Model file for the job. Use its own axes, mm. A direction names the side the tool comes from. Round coordinates to 2 decimals unless told otherwise and drop trailing zeros. Loops run counter-clockwise (first coordinate to the right, second up) from the corner with the lowest first, then second, coordinate; pieces in that order, holes last. Notation, with made-up numbers: M 32.5,49.25 L 82.5,49.25 A29 ccw 82.5,85.25 Z; hole C 2.25,19.5 d6. An arc over 180 degrees is marked long. Use a Markdown table: item, result. Add a question column.
Q1. Mould opens along X. For faces 1 (the face through (-10.867, 76.095, 2.958)), 2 (the face through (-3, 4, 3)), 3 (the face through (-10, 46, 0)) say: +X half, -X half, draft (parallel to the pull), parting line (faces both ways), or undercut.
Q2. Cut at D-D (y = 21). Give the cut face in (x, z).
Q3. Cut at B-B (z = 3.75). Give the cut face in (x, y), plus the area to 3 significant figures.
Q4. Tool access for faces 4 (the face through (-10, 46, 6)), 5 (the face through (-2, 8, 3)), 6 (the face through (-3, 58, 3)): list every direction of +Z, -Z, +X, -X, +Y, -Y with a clear straight run to the whole face (end or side of a thin tool).
Q5. Probe line 1 (Y direction, x = -7.5, z = 4.35); line 2 (X direction, y = 23, z = 3.8); line 3 (X direction, y = 79, z = 1.6). List the from-to ranges inside material, lowest first. Write a range as from..to.
Q6. Cut at A-A (x = -5). Give the cut face in (y, z), plus the area to 3 significant figures.
Q7. Pin check, flat tips, straight feed: pin 1 (1.8 mm diameter, centred on y = 59, z = 4.5, fed in from +X); pin 2 (3.5 mm diameter, centred on x = -2, z = 3, fed in from -Y); pin 3 (0.9 mm diameter, centred on x = -1, z = 4, fed in from -Y). Stop position of each tip, or through.
Q8. Cut at C-C (x = -10). Give the cut face in (y, z).
from build123d import *

# Parameters (mm, degrees)
ESQUISSE1_R             = 4
ESQUISSE1_W             = 3
ESQUISSE1_H             = 10
BOSS_EXTRU_1_DEPTH      = 6
ENL_V_MAT_EXTRU_1_DEPTH = 6
CONG_1_R                = 10
CONG_2_R                = 20


with BuildPart() as part:
    # Esquisse1 → Boss.-Extru.1 (new body)
    # profile 1 of 4: a face of its own
    with BuildSketch(Plane.XY):
        Polygon((-3, 44), (-3, 54), (-3, 62), (0, 62), (0, 90), (-20, 90), (-20, 0), (-3, 0), (-3, 8), (-3, 18), (-3, 26), (-3, 36), align=None)
        with Locations((-10, 80)):
            Circle(ESQUISSE1_R, mode=Mode.SUBTRACT)
    # profile 2 of 4: a face of its own
    with BuildSketch(Plane.XY):
        with Locations((-1.5, 49)):
            Rectangle(ESQUISSE1_W, ESQUISSE1_H)
    # profile 3 of 4: a face of its own
    with BuildSketch(Plane.XY):
        with Locations((-1.5, 31)):
            Rectangle(ESQUISSE1_W, ESQUISSE1_H)
    # profile 4 of 4: a face of its own
    with BuildSketch(Plane.XY):
        with Locations((-1.5, 13)):
            Rectangle(ESQUISSE1_W, ESQUISSE1_H)
    extrude(amount=BOSS_EXTRU_1_DEPTH)

    # Esquisse2 → Enlèv. mat.-Extru.1 (cut)
    with BuildSketch(Plane.XY.offset(6)):
        Polygon((-3, 62), (-8, 62), (-8, 70), (0, 70), (0, 62), align=None)
    extrude(amount=-ENL_V_MAT_EXTRU_1_DEPTH, mode=Mode.SUBTRACT)

    # Congé1
    # the kernel refuses this fillet: 10 mm, written as the material it takes off along each edge
    with BuildSketch(Plane(origin=(-20, 90, -25), x_dir=(0, -1, 0), z_dir=(0, 0, 1)), Plane(origin=(0, 90, -25), x_dir=(-1, 0, 0), z_dir=(0, 0, 1))) as cong_1_piece_1:
        with BuildLine():
            CenterArc((CONG_1_R, CONG_1_R), CONG_1_R, 180, 90)
            Line((0, CONG_1_R), (-CONG_1_R * 0.02, CONG_1_R))
            Line((-CONG_1_R * 0.02, CONG_1_R), (-CONG_1_R * 0.02, -CONG_1_R * 0.02))
            Line((-CONG_1_R * 0.02, -CONG_1_R * 0.02), (CONG_1_R, -CONG_1_R * 0.02))
            Line((CONG_1_R, -CONG_1_R * 0.02), (CONG_1_R, 0))
        make_face()
    extrude(amount=56, mode=Mode.SUBTRACT)
    with BuildSketch(Plane(origin=(0, 70, 30.494897428), x_dir=(0, 1, 0), z_dir=(0, 0, -1))) as cong_1_piece_2:
        with BuildLine():
            CenterArc((9.797958971, -10), CONG_1_R, 90, 78.463040967)
            Line((0, -8), (-0.195959179, -7.96))
            ThreePointArc((-0.195959179, -7.96), (-0.2, -4), (-0.2, 0))
            Line((-0.2, 0), (0, 0.2))
            Line((0, 0.2), (9.797958971, 0.2))
            Line((9.797958971, 0.2), (9.797958971, 0))
        make_face()
    extrude(amount=54.989794856, mode=Mode.SUBTRACT)

    # Congé2
    # the kernel refuses this fillet: 20 mm, written as the material it takes off along each edge
    with BuildSketch(Plane(origin=(-20, 0, -49.434299833), x_dir=(1, 0, 0), z_dir=(0, 0, 1))) as cong_2_piece_1:
        with BuildLine():
            CenterArc((20, 19.773719933), CONG_2_R, 180, 81.373073441)
            Line((0, 19.773719933), (-0.4, 19.773719933))
            Line((-0.4, 19.773719933), (-0.4, 0))
            Line((-0.4, 0), (0, -0.4))
            ThreePointArc((0, -0.4), (8.5, -0.4), (16.94, -0.395474399))
            Line((16.94, -0.395474399), (17, 0))
        make_face()
    extrude(amount=104.868599666, mode=Mode.SUBTRACT)


solid = part.part
Checked values:
| question | item | result |
|---|---|---|
| 1 | face 1 | undercut |
| 1 | face 2 | +X half |
| 1 | face 3 | draft |
| 2 | outline | M -20,0 L -3,0 L -3,6 L -20,6 Z |
| 3 | outline | M -20,19.77 A20 ccw -3,0 L -3,8 L 0,8 L 0,18 L -3,18 L -3,26 L 0,26 L 0,36 L -3,36 L -3,44 L 0,44 L 0,54 L -3,54 L -3,62 L -8,62 L -8,70 A10 ccw 0,79.8 L 0,80 A10 ccw -20,80 Z; hole C -10,80 d8 |
| 3 | area | 1,450 mm^2 |
| 4 | face 4 | +Z, +X, -X, +Y, -Y |
| 4 | face 5 | +Z, -Z, +X, -Y |
| 4 | face 6 | +Z, -Z, +X |
| 5 | line 1 | y = 1.23..62, 70.12..76.88, 83.12..89.68 |
| 5 | line 2 | x = -20..-3 |
| 5 | line 3 | x = -20..-13.87, -6.13..-0.03 |
| 6 | outline | M 0.41,0 L 62,0 L 62,6 L 0.41,6 Z; M 71.14,0 L 88.66,0 L 88.66,6 L 71.14,6 Z |
| 6 | area | 475 mm^2 |
| 7 | pin 1 | stops at x = -3 |
| 7 | pin 2 | stops at y = 0 |
| 7 | pin 3 | stops at y = 8 |
| 8 | outline | M 2.45,0 L 76,0 L 76,6 L 2.45,6 Z; M 84,0 L 90,0 L 90,6 L 84,6 Z |
